Here's how the part is built. I have some questions about the finished solid (model axes, mm). Face numbers are marked on the shaded views. A direction names the side the tool comes from. Round coordinates to 2 decimals unless told otherwise and drop trailing zeros. Loops run counter-clockwise (first coordinate to the right, second up) from the corner with the lowest first, then second, coordinate; pieces in that order, holes last. Notation, with made-up numbers: M 52,-18 L 110,-18 A24 ccw 110,19 Z; hole C -4.5,86 d9. An arc over 180 degrees is marked long. Answer as a JSON object with one key per item and string values.
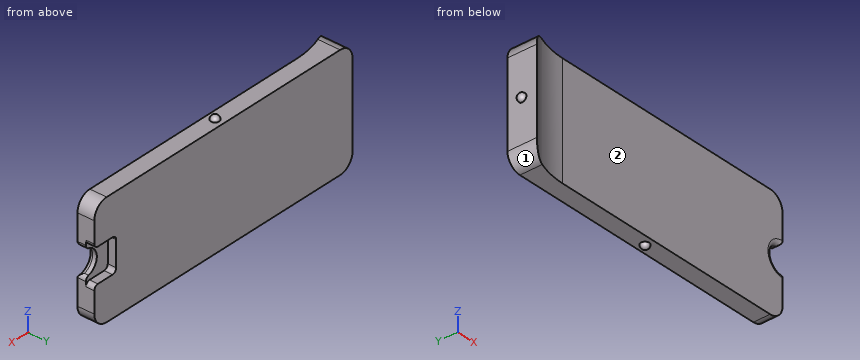
from build123d import *

# Parameters (mm, degrees)
AUFSATZ_LINEAR_AUSTRAGEN1_DEPTH = 6
SCHNITT_LINEAR_AUSTRAGEN1_DEPTH = 39.601165786
SKIZZE5_R                       = 1.5
SCHNITT_LINEAR_AUSTRAGEN2_DEPTH = 39.472457686
SKIZZE6_W                       = 3
SKIZZE6_H                       = 4
SCHNITT_LINEAR_AUSTRAGEN3_DEPTH = 1
VERRUNDUNG2_R                   = 0.5


with BuildPart() as part:
    # Skizze1 → Aufsatz-Linear austragen1 (new body)
    with BuildSketch(Plane(origin=(0, 0, 0), x_dir=(1, 0, 0), z_dir=(0, 1, 0))):
        with BuildLine():
            Line((2, 0.3), (34, 0.3))
            ThreePointArc((34, 0.3), (35.202081528, 0.797918472), (35.7, 2))
            Line((35.7, 2), (35.7, 12))
            ThreePointArc((35.7, 12), (35.202081528, 13.202081528), (34, 13.7))
            Line((34, 13.7), (2, 13.7))
            ThreePointArc((2, 13.7), (0.797918472, 13.202081528), (0.3, 12))
            Line((0.3, 12), (0.3, 2))
            ThreePointArc((0.3, 2), (0.797918472, 0.797918472), (2, 0.3))
        make_face()
    extrude(amount=AUFSATZ_LINEAR_AUSTRAGEN1_DEPTH)

    # Skizze2 → Schnitt-Linear austragen1 (cut, through all)
    with BuildSketch(Plane(origin=(0, 0, -13.7), x_dir=(-1, 0, 0), z_dir=(0, 0, -1))):
        with BuildLine():
            Line((-35.7, 0), (2.436435526, 0))
            ThreePointArc((2.436435526, 0), (-1.091428519, 2.94427191), (-5.563564474, 4))
            Line((-5.563564474, 4), (-35.7, 4))
            Line((-35.7, 4), (-35.7, 0))
        make_face()
    extrude(amount=-SCHNITT_LINEAR_AUSTRAGEN1_DEPTH, mode=Mode.SUBTRACT)

    # Skizze3 → Rotation1 (revolve)
    with BuildSketch(Plane(origin=(0, 0, -13.7), x_dir=(-1, 0, 0), z_dir=(0, 0, -1))):
        with BuildLine():
            Line((-18.5, 5), (-17.5, 5))
            ThreePointArc((-17.5, 5), (-18, 5.5), (-18.5, 5))
        make_face()
    rotation1 = revolve(axis=Axis((35.7, 5, -13.7), (-1, 0, 0)))

    # Skizze4 → Rotation2 (revolve)
    with BuildSketch(Plane.ZY.offset(-0.3)):
        with BuildLine():
            Line((-7, 3.75132006), (-7, 4.75132006))
            ThreePointArc((-7, 4.75132006), (-7.5, 4.25132006), (-7, 3.75132006))
        make_face()
    revolve(axis=Axis((0.3, 2.502640121, -7), (0, 1, 0)))

    # Spiegeln1: Rotation1 across plane
    add(rotation1.mirror(Plane(origin=(0, 0, -7), x_dir=(1, 0, 0), z_dir=(0, 0, -1))))

    # Skizze5 → Schnitt-Linear austragen2 (cut, through all)
    with BuildSketch(Plane.XZ.offset(-4)):
        with Locations((35.7, -7)):
            Circle(SKIZZE5_R)
    extrude(amount=-SCHNITT_LINEAR_AUSTRAGEN2_DEPTH, mode=Mode.SUBTRACT)

    # Skizze6 → Schnitt-Linear austragen3 (cut)
    with BuildSketch(Plane(origin=(0, 6, 0), x_dir=(1, 0, 0), z_dir=(0, 1, 0))):
        with Locations((34.2, 7)):
            Rectangle(SKIZZE6_W, SKIZZE6_H)
    extrude(amount=-SCHNITT_LINEAR_AUSTRAGEN3_DEPTH, mode=Mode.SUBTRACT)

    # Verrundung2
    verrundung2_edges = [part.edges().sort_by_distance(p)[0] for p in [
        (34.2, 4, -7),
        (35.7, 4.5, -5.5),
        (35.7, 4.5, -8.5),
        (35.7, 5.5, -9),
        (35.7, 5.5, -5),
        (32.7, 5.5, -5),
        (32.7, 5.5, -9),
    ]]
    fillet(verrundung2_edges, radius=VERRUNDUNG2_R)


solid = part.part
Item 1: I want a section at A-A, the plane x = 22. Please give me the cut outline in (y, z), then the cut area to 3 significant figures.
Resolved:
{"outline": "M 4,-13.7 L 6,-13.7 L 6,-0.3 L 4,-0.3 Z", "area": "26.8 mm²"}
Item 2: On a 3-axis mill with a long thin cutter (end or side, diameter ignored), from which of +Z, -Z, +X, -X, +Y, -Y can I reach the whole of each face in a straight line? I mean the marked faces 1 and 2. Say none if no direction works.
Resolved:
{"face 1": "-Z, -X, +Y, -Y", "face 2": "+Z, -Z, +X, -Y"}
Item 3: I want a section at C-C, the plane y = 2.9. Please give me the cut outline in (x, z).
Resolved:
{"outline": "M 0.3,-12 A1.7 ccw 1,-13.38 L 1,-0.62 A1.7 ccw 0.3,-2 Z"}
Item 4: I'm going to push flat-ended pins straight in: pin 1 Ø6.5 at (x, z) = (18.5, -7.5) entering from -Y; pin 2 Ø1.1 at (x, y) = (34, 5.5) entering from -Z; pin 3 Ø1.5 at (y, z) = (4.5, -10.5) entering from -X. Where does each tip first touch, or does it pass through?
Resolved:
{"pin 1": "y = 4", "pin 2": "z = -13.7", "pin 3": "x = 0.3"}
Item 5: I want a section at B-B, the plane z = -10. Please give me the cut outline in (x, y), then the cut area to 3 significant figures.
Resolved:
{"outline": "M 0.3,2.5 A10 cw 5.56,4 L 35.7,4 L 35.7,6 L 0.3,6 Z", "area": "73.3 mm²"}
Item 6: Please list where these lines run through material, in increasing order: probe 1 along Y at (x, z) = (11, -3); probe 2 along Z at (x, y) = (26, 5.65); probe 3 along X at (y, z) = (5.8, -10.25). Write a range as from..to.
Resolved:
{"probe 1": "4..6", "probe 2": "-13.7..-0.3", "probe 3": "0.3..35.7"}
